Geometry: final body of the model. Coordinates: model frame, mm. Face numbers are marked on the shaded views. A direction names the side the tool comes from. Give positions to 0.01 mm unless a question says otherwise; leave off trailing zeros. Write each loop counter-clockwise with the first axis right and the second up, starting at its lowest first coordinate (ties: lowest second). Pieces come first, ordered by that corner, then holes. Notation, with made-up numbers: (1, -10.75) -> (38, -10.75) arc R12 ccw to (38, 6.25) -> close; hole circle Ø11 at (89, -9.5). An arc over 180 degrees is marked (long way). Use CSV: the item, a comma, the result in double quotes. Start each with the question number.
1) Section B-B (z = -31.65). Output: boundary loops of the cut face in (x, y), plus the area to 3 significant figures.
2) Section C-C (x = 59.38). Output: boundary loops of the cut face in (y, z).
3) Draft query along X for the marked faces 3, 4 and 5. Return one class per face: pulls with the +X half, pulls with the -X half, needs draft (parallel to the pull), parting line crosses it, or undercut.
4) Set-up query: the marked faces 1 and 2. Return all of +Z, -Z, +X, -X, +Y, -Y with unobstructed straight access to the full face (end or side cutting, diameter ignored); none if empty.
5) Section D-D (z = 23.5). Output: boundary loops of the cut face in (x, y), plus the area to 3 significant figures.
6) Contact query for flat-ended pins moving along their axis: P1, Ø17.5, axis at x = -59.38, z = -31.65, coming from the +Y side; P2, Ø1.9, axis at y = -14.5, z = -17.5, coming from the +X side; P3, Ø12.5, axis at x = 59.38, z = 31.65, coming from the -Y side; P4, Ø3, axis at y = -15.5, z = -19.5, coming from the -X side. Output: stop coordinate, or through.
7) Section A-A (y = -5.5). Output: boundary loops of the cut face in (x, z), plus the area to 3 significant figures.
8) Material intervals for line 1 (Z direction, x = -59.38, y = -6.25); line 2 (X direction, y = -0.75, z = -29.5); line 3 (X direction, y = -1, z = -19), sorted ascending. Write a range as [from, to].
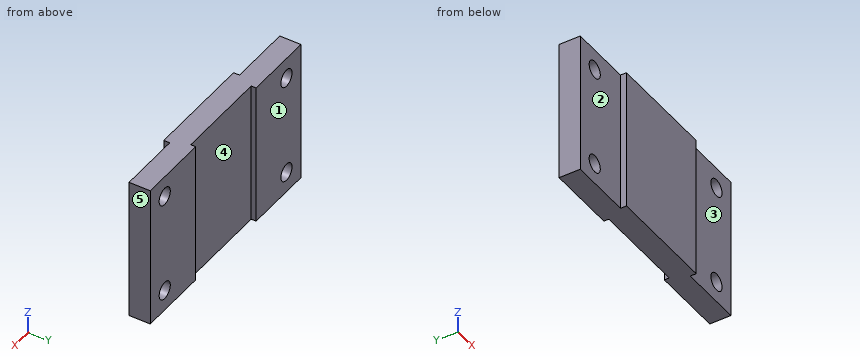
```python
from build123d import *

# Parameters (mm, degrees)
F0_W     = 39.66
F0_H     = 89.64
F0_R     = 5.43
F0_W_2   = 39.22
F1_DEPTH = 13.26
F0_W_3   = 68.06
F2_DEPTH = 16.98
F5_W     = 58.96
F5_H     = 3.08
F6_DEPTH = 89.641


with BuildPart() as f1:
    # F0 (on Front) → F1 (new body)
    with BuildSketch(Plane.XZ):
        with Locations((53.64, 0)):
            Rectangle(F0_W, F0_H)
        with Locations((59.38, -31.65)):
            Circle(F0_R, mode=Mode.SUBTRACT)
        with Locations((59.38, 31.65)):
            Circle(F0_R, mode=Mode.SUBTRACT)
        with Locations((-53.86, 0)):
            Rectangle(F0_W_2, F0_H)
        with Locations((-59.38, -31.65)):
            Circle(F0_R, mode=Mode.SUBTRACT)
        with Locations((-59.38, 31.65)):
            Circle(F0_R, mode=Mode.SUBTRACT)
    extrude(amount=F1_DEPTH)


with BuildPart() as f2:
    # F0 (on Front) → F2 (new body)
    with BuildSketch(Plane.XZ):
        with Locations((-0.22, 0)):
            Rectangle(F0_W_3, F0_H)
    extrude(amount=F2_DEPTH)

    # F3: union F1
    add(f1.part)

    # F4: union 

    # F5 (on face) → F6 (cut, through all)
    with BuildSketch(Plane(origin=(0, 0, -44.82), x_dir=(1, 0, 0), z_dir=(0, 0, -1))):
        Polygon((73.47, -21.704547), (73.47, 0), (29.19, 0), (-29.77, 0), (-73.47, 0), (-73.47, -21.704547), align=None)
        with Locations((-0.29, 1.54)):
            Rectangle(F5_W, F5_H)
    extrude(amount=-F6_DEPTH, mode=Mode.SUBTRACT)


solid = f2.part
```
Answers follow:
1,outline,"(-73.47, -13.26) -> (-64.81, -13.26) -> (-64.81, 0) -> (-73.47, 0) -> close; (-53.95, -13.26) -> (-34.25, -13.26) -> (-34.25, -16.98) -> (33.81, -16.98) -> (33.81, -13.26) -> (53.95, -13.26) -> (53.95, 0) -> (29.19, 0) -> (29.19, -3.08) -> (-29.77, -3.08) -> (-29.77, 0) -> (-53.95, 0) -> close; (64.81, -13.26) -> (73.47, -13.26) -> (73.47, 0) -> (64.81, 0) -> close"
1,area,"1,730 mm^2"
2,outline,"(-13.26, -44.82) -> (0, -44.82) -> (0, -37.08) -> (-13.26, -37.08) -> close; (-13.26, -26.22) -> (0, -26.22) -> (0, 26.22) -> (-13.26, 26.22) -> close; (-13.26, 37.08) -> (0, 37.08) -> (0, 44.82) -> (-13.26, 44.82) -> close"
3,face 3,"needs draft"
3,face 4,"undercut"
3,face 5,"pulls with the +X half"
4,face 1,"+Z, -Z, +X, -X, +Y"
4,face 2,"+Z, -Z, -X, -Y"
5,outline,"(-73.47, -13.26) -> (-34.25, -13.26) -> (-34.25, -16.98) -> (33.81, -16.98) -> (33.81, -13.26) -> (73.47, -13.26) -> (73.47, 0) -> (29.19, 0) -> (29.19, -3.08) -> (-29.77, -3.08) -> (-29.77, 0) -> (-73.47, 0) -> close"
5,area,"2,020 mm^2"
6,P1,"stops at y = 0"
6,P2,"stops at x = 33.81"
6,P3,"stops at y = -13.26"
6,P4,"stops at x = -34.25"
7,outline,"(-73.47, -44.82) -> (73.47, -44.82) -> (73.47, 44.82) -> (-73.47, 44.82) -> close; hole circle Ø10.86 at (-59.38, -31.65); hole circle Ø10.86 at (-59.38, 31.65); hole circle Ø10.86 at (59.38, -31.65); hole circle Ø10.86 at (59.38, 31.65)"
7,area,"12,800 mm^2"
8,line 1,"z = [-44.82, -37.08], [-26.22, 26.22], [37.08, 44.82]"
8,line 2,"x = [-73.47, -64.37], [-54.39, -29.77], [29.19, 54.39], [64.37, 73.47]"
8,line 3,"x = [-73.47, -29.77], [29.19, 73.47]"
